Geometry check sheet. Reference: the model listing, model coordinates, mm. Coordinates: 2 decimals unless noted, no trailing zeros. Order: outer loops, then holes, each group sorted by start corner. A loop starts at its lowest first (then second) coordinate and runs counter-clockwise, first axis right, second up. Notation, with made-up numbers: (75.25, 17.5) -> (86.25, 17.5) arc R7 ccw to (86.25, 23.5) -> close; hole circle Ø4 at (46, -25.5). An arc over 180 degrees is marked (long way). Answer in a Markdown table with one row per item. Add a question column.
```python
from build123d import *

# Parameters (mm, degrees)
PAD_DEPTH         = 1500
SKETCH004_R       = 4
POCKET003_DEPTH   = 50.001
SKETCH005_R       = 6.5
POCKET004_DEPTH   = 50.001
SKETCH006_R       = 6.5
POCKET_DEPTH      = 50.001
POCKET_DEPTH_BACK = -50.001


with BuildPart() as part:
    # Sketch → Pad (new body)
    with BuildSketch(Plane.YZ):
        with BuildLine():
            Line((-45, 50), (45, 50))
            ThreePointArc((50, 45), (48.535534, 48.535534), (45, 50))
            Line((50, 45), (50, -45))
            ThreePointArc((45, -50), (48.535534, -48.535534), (50, -45))
            Line((45, -50), (-45, -50))
            ThreePointArc((-50, -45), (-48.535534, -48.535534), (-45, -50))
            Line((-50, -45), (-50, 45))
            ThreePointArc((-45, 50), (-48.535534, 48.535534), (-50, 45))
        make_face()
        with BuildLine():
            Line((-40, 45), (40, 45))
            ThreePointArc((45, 40), (43.535534, 43.535534), (40, 45))
            Line((45, 40), (45, -40))
            ThreePointArc((40, -45), (43.535534, -43.535534), (45, -40))
            Line((40, -45), (-40, -45))
            ThreePointArc((-45, -40), (-43.535534, -43.535534), (-40, -45))
            Line((-45, -40), (-45, 40))
            ThreePointArc((-40, 45), (-43.535534, 43.535534), (-45, 40))
        make_face(mode=Mode.SUBTRACT)
    extrude(amount=PAD_DEPTH)

    # Sketch004 → Pocket003 (cut, through all)
    with BuildSketch(Plane.XZ):
        with Locations((880.218, 24)):
            Circle(SKETCH004_R)
        with Locations((880.218, -24)):
            Circle(SKETCH004_R)
        with Locations((820.218, 24.000003)):
            Circle(SKETCH004_R)
        with Locations((760.218, 24.000007)):
            Circle(SKETCH004_R)
        with Locations((700.218, 24.00001)):
            Circle(SKETCH004_R)
        with Locations((640.218, 24.000014)):
            Circle(SKETCH004_R)
        with Locations((580.218, 24.000017)):
            Circle(SKETCH004_R)
        with Locations((520.218, 24.00002)):
            Circle(SKETCH004_R)
        with Locations((460.218, 24.000024)):
            Circle(SKETCH004_R)
        with Locations((400.218, 24.000027)):
            Circle(SKETCH004_R)
        with Locations((340.218, 24.000031)):
            Circle(SKETCH004_R)
        with Locations((280.218, 24.000034)):
            Circle(SKETCH004_R)
        with Locations((220.218, 24.000037)):
            Circle(SKETCH004_R)
        with Locations((160.218, 24.000041)):
            Circle(SKETCH004_R)
        with Locations((100.218, 24.000044)):
            Circle(SKETCH004_R)
        with Locations((820.218, -24.000003)):
            Circle(SKETCH004_R)
        with Locations((760.218, -24.000006)):
            Circle(SKETCH004_R)
        with Locations((700.218, -24.000009)):
            Circle(SKETCH004_R)
        with Locations((640.218, -24.000012)):
            Circle(SKETCH004_R)
        with Locations((580.218, -24.000015)):
            Circle(SKETCH004_R)
        with Locations((520.218, -24.000018)):
            Circle(SKETCH004_R)
        with Locations((460.218, -24.000021)):
            Circle(SKETCH004_R)
        with Locations((400.218, -24.000023)):
            Circle(SKETCH004_R)
        with Locations((340.218, -24.000026)):
            Circle(SKETCH004_R)
        with Locations((280.218, -24.000029)):
            Circle(SKETCH004_R)
        with Locations((220.218, -24.000032)):
            Circle(SKETCH004_R)
        with Locations((160.218, -24.000035)):
            Circle(SKETCH004_R)
        with Locations((100.218, -24.000038)):
            Circle(SKETCH004_R)
    extrude(amount=-POCKET003_DEPTH, mode=Mode.SUBTRACT)

    # Sketch005 → Pocket004 (cut, through all)
    with BuildSketch(Plane.XZ):
        with Locations((12, 24)):
            Circle(SKETCH005_R)
        with Locations((12, -24)):
            Circle(SKETCH005_R)
        with Locations((1460, 0)):
            Circle(SKETCH005_R)
    extrude(amount=POCKET004_DEPTH, mode=Mode.SUBTRACT)

    # Sketch006 → Pocket (cut, two sides)
    with BuildSketch(Plane.XY) as pocket_sk:
        with Locations((35, 24)):
            Circle(SKETCH006_R)
        with Locations((35, -24)):
            Circle(SKETCH006_R)
        with Locations((85, 24)):
            Circle(SKETCH006_R)
        with Locations((135, 24)):
            Circle(SKETCH006_R)
        with Locations((135, -24)):
            Circle(SKETCH006_R)
        with Locations((85, -24)):
            Circle(SKETCH006_R)
        with Locations((442.5, 24)):
            Circle(SKETCH006_R)
        with Locations((442.5, -24)):
            Circle(SKETCH006_R)
        with Locations((750, 24)):
            Circle(SKETCH006_R)
        with Locations((750, -24)):
            Circle(SKETCH006_R)
        with Locations((1057.5, 24)):
            Circle(SKETCH006_R)
        with Locations((1057.5, -24)):
            Circle(SKETCH006_R)
        with Locations((1365, 24)):
            Circle(SKETCH006_R)
        with Locations((1415, 24)):
            Circle(SKETCH006_R)
        with Locations((1465, 24)):
            Circle(SKETCH006_R)
        with Locations((1465, -24)):
            Circle(SKETCH006_R)
        with Locations((1415, -24)):
            Circle(SKETCH006_R)
        with Locations((1365, -24)):
            Circle(SKETCH006_R)
        with Locations((1297.5, 24)):
            Circle(SKETCH006_R)
        with Locations((1217.5, 24)):
            Circle(SKETCH006_R)
        with Locations((1137.5, 24)):
            Circle(SKETCH006_R)
    extrude(amount=-POCKET_DEPTH, mode=Mode.SUBTRACT)
    extrude(pocket_sk.sketch, amount=-POCKET_DEPTH_BACK, mode=Mode.SUBTRACT)


solid = part.part
```
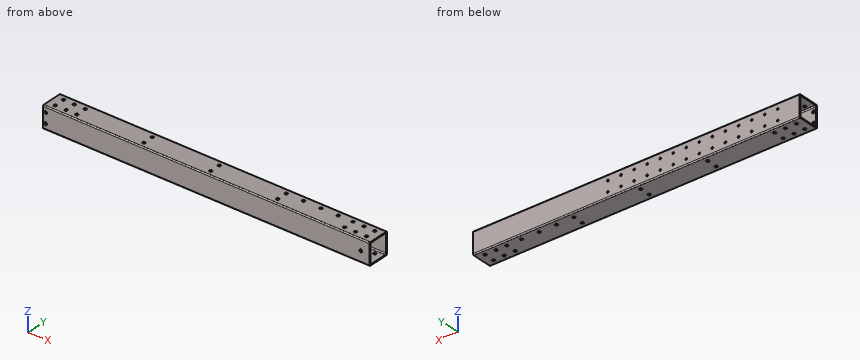
(1) Go/stop test with flat-tipped pins: P1, Ø7, axis at x = 580.22, z = 24, coming from the +Y side; P2, Ø8, axis at x = 1415, y = -24, coming from the -Z side. Record where each tip stops, or that it passes through.
(2) Scan lines: line 1 along Z through (x, y) = (959.5, -0.5); line 2 along Y through (x, z) = (280, -22.5). Record each from-to range of solid material in increasing order.
(3) Cross-section at A-A (y = 0). Enter the section's corners in (x, z).
Checks:
| question | item | result |
|---|---|---|
| 1 | P1 | y = -45 |
| 1 | P2 | through |
| 2 | line 1 | -50 to -45, 45 to 50 |
| 2 | line 2 | -50 to -45 |
| 3 | outline | (0, -50) -> (1500, -50) -> (1500, -45) -> (0, -45) -> close; (0, 45) -> (1500, 45) -> (1500, 50) -> (0, 50) -> close |
